Can you work these out from the model? Positions are in its coordinate system, mm. A direction names the side the tool comes from. Coordinates: 2 decimals unless noted, no trailing zeros. Loops run counter-clockwise (first coordinate to the right, second up) from the corner with the lowest first, then second, coordinate; pieces in that order, holes last.
```python
from build123d import *

# Parameters (mm, degrees)
SKETCH1_W           = 7
SKETCH1_H           = 5
BOSS_EXTRUDE1_DEPTH = 30
SKETCH3_W           = 1
SKETCH3_H           = 5
CUT_EXTRUDE1_DEPTH  = 10
SKETCH4_W           = 4
SKETCH4_H           = 5
CUT_EXTRUDE2_DEPTH  = 18
CUT_EXTRUDE3_REACH  = 7
CUT_EXTRUDE5_DEPTH  = 8
SKETCH8_R           = 0.5
CUT_EXTRUDE6_DEPTH  = 8
SKETCH9_R           = 1
CUT_EXTRUDE7_DEPTH  = 10


with BuildPart() as part:
    # Sketch1 → Boss-Extrude1 (new body)
    with BuildSketch(Plane(origin=(0, 0, 0), x_dir=(1, 0, 0), z_dir=(0, 1, 0))):
        Rectangle(SKETCH1_W, SKETCH1_H)
    extrude(amount=BOSS_EXTRUDE1_DEPTH)

    # Sketch3 → Cut-Extrude1 (cut)
    with BuildSketch(Plane.XZ):
        with Locations((-3, 0)):
            Rectangle(SKETCH3_W, SKETCH3_H)
        with Locations((3, 0)):
            Rectangle(SKETCH3_W, SKETCH3_H)
    extrude(amount=-CUT_EXTRUDE1_DEPTH, mode=Mode.SUBTRACT)

    # Sketch4 → Cut-Extrude2 (cut)
    with BuildSketch(Plane(origin=(0, 30, 0), x_dir=(1, 0, 0), z_dir=(0, 1, 0))):
        Rectangle(SKETCH4_W, SKETCH4_H)
    extrude(amount=-CUT_EXTRUDE2_DEPTH, mode=Mode.SUBTRACT)

    # Sketch5 → Cut-Extrude3 (cut, up to next)
    with BuildSketch(Plane.XY.offset(2.5), mode=Mode.PRIVATE) as cut_extrude3_sk1:
        Polygon((-3.5, 10), (-2.5, 10), (-3.5, 11), align=None)
    cut_extrude3_tool1 = extrude(cut_extrude3_sk1.sketch, amount=-CUT_EXTRUDE3_REACH, mode=Mode.PRIVATE) & part.part
    add(cut_extrude3_tool1.solids().sort_by_distance((-3.166667, 10.333333, 2.5))[0], mode=Mode.SUBTRACT)
    # Sketch5 → Cut-Extrude3 (cut, up to next)
    with BuildSketch(Plane.XY.offset(2.5), mode=Mode.PRIVATE) as cut_extrude3_sk2:
        Polygon((3.5, 11), (3.5, 10), (2.5, 10), align=None)
    cut_extrude3_tool2 = extrude(cut_extrude3_sk2.sketch, amount=-CUT_EXTRUDE3_REACH, mode=Mode.PRIVATE) & part.part
    add(cut_extrude3_tool2.solids().sort_by_distance((3.166667, 10.333333, 2.5))[0], mode=Mode.SUBTRACT)

    # Sketch7 → Cut-Extrude5 (cut, through all)
    with BuildSketch(Plane(origin=(3.5, 0, 0), x_dir=(0, 0, -1), z_dir=(1, 0, 0))):
        with BuildLine():
            Line((-2.5, 27.5), (-2.5, 30))
            Line((-2.5, 30), (2.5, 30))
            Line((2.5, 30), (2.5, 27.5))
            ThreePointArc((2.5, 27.5), (1.756951521, 29.241656191), (0, 29.947778476))
            ThreePointArc((0, 29.947778476), (-1.756951521, 29.241656191), (-2.5, 27.5))
        make_face()
    extrude(amount=-CUT_EXTRUDE5_DEPTH, mode=Mode.SUBTRACT)

    # Sketch8 → Cut-Extrude6 (cut, through all)
    with BuildSketch(Plane(origin=(3.5, 0, 0), x_dir=(0, 0, -1), z_dir=(1, 0, 0))):
        with Locations((0, 27.5)):
            Circle(SKETCH8_R)
    extrude(amount=-CUT_EXTRUDE6_DEPTH, mode=Mode.SUBTRACT)

    # Sketch9 → Cut-Extrude7 (cut)
    with BuildSketch(Plane.XZ):
        Circle(SKETCH9_R)
    extrude(amount=-CUT_EXTRUDE7_DEPTH, mode=Mode.SUBTRACT)


solid = part.part
```
(1) I want a section at C-C on z = -1.8. Write out the boundary of the cut face in (x, y), then the cut area to 3 significant figures.
Check values:
outline: (-3.5, 11) - (-2.5, 10) - (-2.5, 0) - (2.5, 0) - (2.5, 10) - (3.5, 11) - (3.5, 29.2) - (2, 29.2) - (2, 12) - (-2, 12) - (-2, 29.2) - (-3.5, 29.2) - close
area: 115 mm2
(2) If I drill on probe 1 along X at (y, z) = (27.5, -1.25); probe 2 along Z at (x, y) = (0, 2); probe 3 along Y at (x, z) = (-2.65, 0), over which ranges is the centre line in solid material (lowest first)?
Check values:
probe 1: x = -3.5 to -2, 2 to 3.5
probe 2: z = -2.5 to -1, 1 to 2.5
probe 3: y = 10.15 to 27, 28 to 29.95
(3) I want a section at A-A on x = 0. Write out the boundary of the cut face in (y, z), then the cut area to 3 significant figures.
Check values:
outline: (0, -2.5) - (12, -2.5) - (12, 2.5) - (0, 2.5) - (0, 1) - (10, 1) - (10, -1) - (0, -1) - close
area: 40.0 mm2
(4) I'm going to push flat-ended pins straight in: pin 1 (1.5 mm diameter, centred on y = 3.5, z = 0.5, fed in from +X); pin 2 (1.2 mm diameter, centred on x = 0.5, z = 1, fed in from +Y). Where does each tip first touch, or does it pass through?
Check values:
pin 1: stops at x = 2.5
pin 2: stops at y = 12
(5) Which directions (+Z, -Z, +X, -X, +Y, -Y) give clear straight access to the entire face, cutting with the end or side of a thin tool? Please do faces 1 (the flat face through (-2.5, 5, 0)), 2 (the flat face through (0, 10, 0)), 3 (the flat face through (2, 21, 0)).
Check values:
face 1: +Z, -Z, -X, -Y
face 2: -Y
face 3: +Z, -Z, +Y
(6) If we mould it in two halves opening along X, with no side actions, what happens to faces 4 (the cylindrical face through (0, 5, -1)), 5 (the flat face through (3, 10.5, 0)), 6 (the cylindrical face through (3, 28, 0))? For each: released by +X, released by -X, zero draft, split by the parting line, or undercut.
Check values:
face 4: undercut
face 5: released by +X
face 6: zero draft
(7) I want a section at B-B on y = 16. Write out the boundary of the cut face in (x, z).
Check values:
outline: (-3.5, -2.5) - (-2, -2.5) - (-2, 2.5) - (-3.5, 2.5) - close; (2, -2.5) - (3.5, -2.5) - (3.5, 2.5) - (2, 2.5) - close
